Here's how the part is built. I have some questions about the finished solid (model axes, mm). A direction names the side the tool comes from. Coordinates: 2 decimals unless noted, no trailing zeros. Write each loop counter-clockwise with the first axis right and the second up, starting at its lowest first coordinate (ties: lowest second). Pieces come first, ordered by that corner, then holes.
Item 1: If we mould it in two halves opening along X, with no side actions, what happens to faces 1 (the face through (9.824, 2.465, -16.748)), 2 (the face through (20, 6, -14)), 3 (the face through (0, 6, -14)), 4 (the face through (10, 6, -20))? For each: pulls with the +X half, pulls with the -X half, needs draft (parallel to the pull), parting line crosses it, or undercut.
Item 2: I want a section at B-B (z = -11). Please give me the cut outline in (x, y).
Item 3: I want a section at D-D (z = -15.25). Please give me the cut outline in (x, y), and give its area (3 significant figures).
Item 4: I want a section at C-C (y = 7.75). Please give me the cut outline in (x, z).
Item 5: I want a section at A-A (x = 10). Please give me the cut outline in (y, z), and give its area (4 significant figures).
Item 6: For faces 5 (the face through (10, 11, -15)), 6 (the face through (9.87, 7.96, -14.75)), 7 (the face through (10, 5, -15)), which set-ups out of +Z, -Z, +X, -X, +Y, -Y let a thin tool reach every point of the face, with its end or its side?
Item 7: I'm going to push flat-ended pins straight in: P1, Ø2.5, axis at x = 9.5, z = -11.5, coming from the +Y side; P2, Ø1.5, axis at x = 14.5, z = -14, coming from the +Y side. Where does each tip first touch, or does it pass through?
Item 8: Please list where these lines run through material, in increasing order: line 1 (X direction, y = 7, z = -14.25); line 2 (Y direction, x = 3.5, z = -11); line 3 (X direction, y = 3, z = -15.5).
from build123d import *

# Parameters (mm, degrees)
EXTRUDE_1_DEPTH = 5
EXTRUDE_2_DEPTH = 6
EXTRUDE_3_DEPTH = 2


with BuildPart() as part:
    # 草图1 → 凸台-拉伸1 (new body)
    with BuildSketch(Plane(origin=(0, 0, 0), x_dir=(1, 0, 0), z_dir=(0, 1, 0))):
        with BuildLine():
            Line((0, 8.75), (2, 8.75))
            ThreePointArc((2, 8.75), (10, 16.75), (18, 8.75))
            Line((18, 8.75), (20, 8.75))
            Line((20, 8.75), (20, 20))
            Line((20, 20), (0, 20))
            Line((0, 20), (0, 8.75))
        make_face()
    extrude(amount=EXTRUDE_1_DEPTH)

    # 草图2 → 凸台-拉伸2 (add)
    with BuildSketch(Plane(origin=(0, 5, 0), x_dir=(1, 0, 0), z_dir=(0, 1, 0))):
        with BuildLine():
            Line((16, 8.75), (20, 8.75))
            Line((20, 8.75), (20, 20))
            Line((20, 20), (0, 20))
            Line((0, 20), (0, 8.75))
            Line((0, 8.75), (4, 8.75))
            ThreePointArc((4, 8.75), (10, 14.75), (16, 8.75))
        make_face()
    extrude(amount=EXTRUDE_2_DEPTH)

    # 草图3 → 凸台-拉伸3 (add)
    with BuildSketch(Plane(origin=(0, 11, 0), x_dir=(1, 0, 0), z_dir=(0, 1, 0))):
        with BuildLine():
            Line((18, 8.75), (20, 8.75))
            Line((20, 8.75), (20, 20))
            Line((20, 20), (0, 20))
            Line((0, 20), (0, 8.75))
            Line((0, 8.75), (2, 8.75))
            ThreePointArc((2, 8.75), (10, 16.75), (18, 8.75))
        make_face()
    extrude(amount=EXTRUDE_3_DEPTH)


solid = part.part
Answer:
1. face 1: undercut
1. face 2: pulls with the +X half
1. face 3: pulls with the -X half
1. face 4: needs draft
2. outline: (0, 0) - (2.32, 0) - (2.32, 5) - (4.44, 5) - (4.44, 11) - (2.32, 11) - (2.32, 13) - (0, 13) - close; (15.56, 5) - (17.68, 5) - (17.68, 0) - (20, 0) - (20, 13) - (17.68, 13) - (17.68, 11) - (15.56, 11) - close
3. outline: (0, 0) - (5.34, 0) - (5.34, 5) - (14.66, 5) - (14.66, 0) - (20, 0) - (20, 13) - (14.66, 13) - (14.66, 11) - (5.34, 11) - (5.34, 13) - (0, 13) - close
3. area: 195 mm2
4. outline: (0, -20) - (20, -20) - (20, -8.75) - (16, -8.75) arc R6 cw to (4, -8.75) - (0, -8.75) - close
5. outline: (0, -20) - (13, -20) - (13, -16.75) - (11, -16.75) - (11, -14.75) - (5, -14.75) - (5, -16.75) - (0, -16.75) - close
5. area: 54.25 mm2
6. face 5: +Z, +Y
6. face 6: +Z, +Y, -Y
6. face 7: +Z, -Y
7. P1: passes through
7. P2: stops at y = 11
8. line 1: x = 0 to 7.6, 12.4 to 20
8. line 2: y = 5 to 11
8. line 3: x = 0 to 5.71, 14.29 to 20
